CAD build for the part. Positions are in the model's coordinates, mm. Give positions to 0.01 mm unless a question says otherwise; leave off trailing zeros. Loops run counter-clockwise (first coordinate to the right, second up) from the corner with the lowest first, then second, coordinate; pieces in that order, holes last. Notation, with made-up numbers: M 34.5,33.5 L 91.5,33.5 A23 cw 91.5,53.5 Z; hole C 35,-30 d11. An arc over 180 degrees is marked long. Answer as CSV lines item,"result".
from build123d import *

# Parameters (mm, degrees)
SKETCH_1_R      = 1.6
SKETCH_1_R_2    = 15
EXTRUDE_1_DEPTH = 3


with BuildPart() as part:
    # 草图1 → 凸台-拉伸1 (new body)
    with BuildSketch(Plane.XY):
        with BuildLine():
            Line((-34, 0), (34, 0))
            Line((34, 0), (34, 40))
            ThreePointArc((34, 40), (33.414213562, 41.414213562), (32, 42))
            Line((32, 42), (-32, 42))
            ThreePointArc((-32, 42), (-33.414213562, 41.414213562), (-34, 40))
            Line((-34, 40), (-34, 0))
        make_face()
        with Locations((15.5, 5.5)):
            Circle(SKETCH_1_R, mode=Mode.SUBTRACT)
        with Locations((-15.5, 5.5)):
            Circle(SKETCH_1_R, mode=Mode.SUBTRACT)
        with Locations((-15.5, 36.5)):
            Circle(SKETCH_1_R, mode=Mode.SUBTRACT)
        with Locations((15.5, 36.5)):
            Circle(SKETCH_1_R, mode=Mode.SUBTRACT)
        with Locations((30, 34)):
            Circle(SKETCH_1_R, mode=Mode.SUBTRACT)
        with Locations((30, 10)):
            Circle(SKETCH_1_R, mode=Mode.SUBTRACT)
        with Locations((-30, 10)):
            Circle(SKETCH_1_R, mode=Mode.SUBTRACT)
        with Locations((-30, 34)):
            Circle(SKETCH_1_R, mode=Mode.SUBTRACT)
        with Locations((0, 21)):
            Circle(SKETCH_1_R_2, mode=Mode.SUBTRACT)
    extrude(amount=EXTRUDE_1_DEPTH)


solid = part.part
1) Mould opens along X. For faces 1 (the face through (33.43, 41.4, 1.48)), 2 (the face through (15.15, 34.94, 1.48)), 3 (the face through (0, 0, 1)) say: +X half, -X half, draft (parallel to the pull), parting line (faces both ways), or undercut.
Answer below:
face 1,"+X half"
face 2,"undercut"
face 3,"draft"
2) Band-saw the part on C-C on x = -30. Give the cut face in (y, z).
Answer below:
outline,"M 0,0 L 8.4,0 L 8.4,3 L 0,3 Z; M 11.6,0 L 32.4,0 L 32.4,3 L 11.6,3 Z; M 35.6,0 L 42,0 L 42,3 L 35.6,3 Z"
3) Band-saw the part on A-A on x = 0. Give the cut face in (y, z), and give its area (3 significant figures).
Answer below:
outline,"M 0,0 L 6,0 L 6,3 L 0,3 Z; M 36,0 L 42,0 L 42,3 L 36,3 Z"
area,"36.0 mm^2"
4) Band-saw the part on D-D on z = 0.7. Give the number of separate pieces and of enclosed holes in the cut face, and give its area (3 significant figures).
Answer below:
separate pieces,"1"
enclosed holes,"9"
area,"2,080 mm^2"
5) Band-saw the part on B-B on y = 21. Give the cut face in (x, z).
Answer below:
outline,"M -34,0 L -15,0 L -15,3 L -34,3 Z; M 15,0 L 34,0 L 34,3 L 15,3 Z"
6) Drill centre lines: line 1 (Y direction, x = 15.5, z = 1.1); line 2 (Y direction, x = 16.5, z = 1.8); line 3 (Y direction, x = 0, z = 0.8). Where is each one in solid material? Low to high. Write a range as from..to.
Answer below:
line 1,"y = 0..3.9, 7.1..34.9, 38.1..42"
line 2,"y = 0..4.25, 6.75..35.25, 37.75..42"
line 3,"y = 0..6, 36..42"
